```python
from build123d import *

# Parameters (mm, degrees)
SKETCH_R          = 20.4
SKETCH_R_2        = 19.2
PAD_DEPTH         = 70
SKETCH001_R       = 1.5
POCKET_DEPTH      = 20.401
POCKET_DEPTH_BACK = -20.401


with BuildPart() as part:
    # Sketch → Pad (new body)
    with BuildSketch(Plane.XY):
        Circle(SKETCH_R)
        Circle(SKETCH_R_2, mode=Mode.SUBTRACT)
    extrude(amount=PAD_DEPTH)

    # Sketch001 → Pocket (cut, two sides)
    with BuildSketch(Plane.XZ) as pocket_sk:
        with Locations((0, 2)):
            Circle(SKETCH001_R)
        with Locations((0, 68)):
            Circle(SKETCH001_R)
    extrude(amount=-POCKET_DEPTH, mode=Mode.SUBTRACT)
    extrude(pocket_sk.sketch, amount=-POCKET_DEPTH_BACK, mode=Mode.SUBTRACT)


solid = part.part
```
Geometry check sheet. Reference: the model listing, model coordinates, mm. Give positions to 0.01 mm unless a question says otherwise; leave off trailing zeros. Write each loop counter-clockwise with the first axis right and the second up, starting at its lowest first coordinate (ties: lowest second). Pieces come first, ordered by that corner, then holes.
1) Section check A-A, the plane y = 0. Record the boundary of the cut face in (x, z).
2) Section check D-D, the plane z = 45.5. Record the boundary of the cut face in (x, y).
3) Section check B-B, the plane x = 0. Record the boundary of the cut face in (y, z), and give its area (3 significant figures).
4) Release check for a two-part mould opening along Y. For faces 1 (the cylindrical face through (10.32, 16.19, 34.51)), 2 (the cylindrical face through (-0.325, -19.762, 0.536)), 3 (the cylindrical face through (9.41, -18.1, 34.51)) record: pulls with the +Y half, pulls with the -Y half, needs draft (parallel to the pull), parting line crosses it, or undercut.
5) Material ranges on L1, parallel to Z at x = 0, y = -19.6; L2, parallel to Y at x = 0, z = 35; L3, parallel to X at y = -0.5, z = 24, recorded low to high.
6) Gauge pin test, flat ends, axial feed: pin 1 (1.5 mm diameter, centred on y = -6, z = 34, fed in from +X); pin 2 (5 mm diameter, centred on x = 4, z = 20, fed in from +Y); pin 3 (2 mm diameter, centred on x = 14, z = 29, fed in from -Y). Record the tip position at first contact, or that the pin passes through.
Computed:
1. outline: (-20.4, 0) - (-19.2, 0) - (-19.2, 70) - (-20.4, 70) - close; (19.2, 0) - (20.4, 0) - (20.4, 70) - (19.2, 70) - close
2. outline: circle Ø40.8 at (0, 0); hole circle Ø38.4 at (0, 0)
3. outline: (-20.4, 0) - (-19.2, 0) - (-19.2, 0.5) - (-20.4, 0.5) - close; (-20.4, 3.5) - (-19.2, 3.5) - (-19.2, 66.5) - (-20.4, 66.5) - close; (-20.4, 69.5) - (-19.2, 69.5) - (-19.2, 70) - (-20.4, 70) - close; (19.2, 0) - (20.4, 0) - (20.4, 0.5) - (19.2, 0.5) - close; (19.2, 3.5) - (20.4, 3.5) - (20.4, 66.5) - (19.2, 66.5) - close; (19.2, 69.5) - (20.4, 69.5) - (20.4, 70) - (19.2, 70) - close
3. area: 154 mm2
4. face 1: undercut
4. face 2: needs draft
4. face 3: parting line crosses it
5. L1: z = 0 to 0.5, 3.5 to 66.5, 69.5 to 70
5. L2: y = -20.4 to -19.2, 19.2 to 20.4
5. L3: x = -20.39 to -19.19, 19.19 to 20.39
6. pin 1: stops at x = 19.71
6. pin 2: stops at y = 20.34
6. pin 3: stops at y = -15.72
